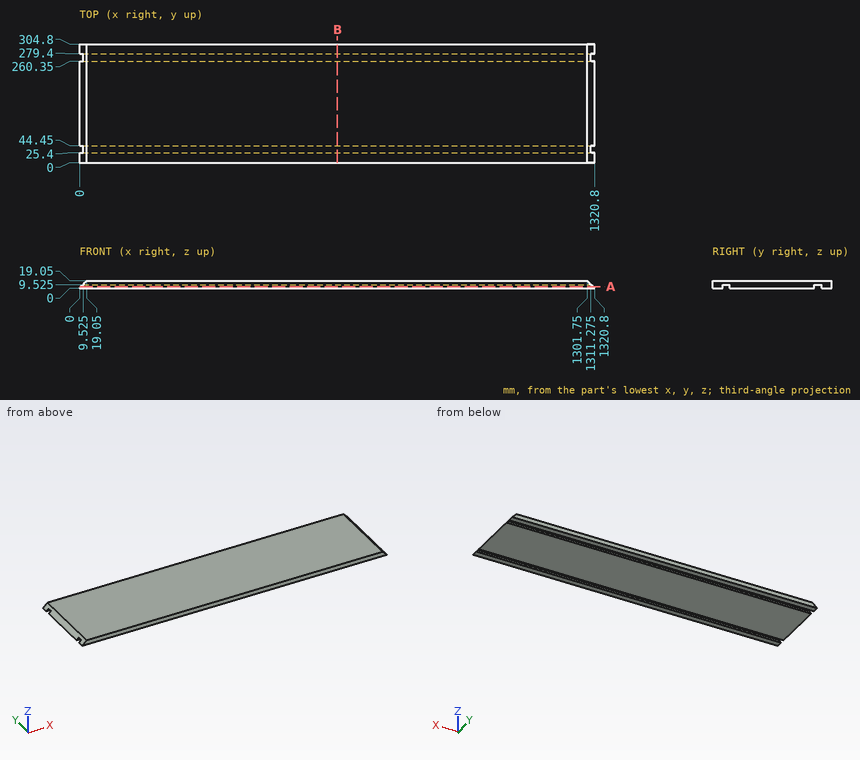
Print and shaded views of the part. All mm, measured from the part's lowest x, y and z. Give positions to 0.01 mm unless a question says otherwise; leave off trailing zeros. Loops run counter-clockwise (first coordinate to the right, second up) from the corner with the lowest first, then second, coordinate; pieces in that order, holes last.
1) Saw through at B-B (x = 661.5). Write the cut outline in (y, z) (3 decimals), plus the area to 3 significant figures.
2) Wall check: line 1 (Y direction, x = 846, z = 1.75); line 2 (X direction, y = 186.5, z = 9.75); line 3 (Z direction, x = 1073.5, y = 39) (3 decimals). Give the ranges that are in metal, low to high.
3) Flat gauge pins, fed straight in: pin 1 Ø3 at (y, z) = (77, 7.5) entering from -X; pin 2 Ø8 at (y, z) = (147.5, 11.5) entering from -X; pin 3 Ø5.5 at (x, y) = (665, 265.5) entering from -Z (3 decimals). Where does each tip first touch, or does it go through?
4) Saw through at A-A (z = 4.25). Write the cut outline in (x, y).
Answer block:
1. outline: (0, 0) - (25.4, 0) - (25.4, 9.525) - (44.45, 9.525) - (44.45, 0) - (260.35, 0) - (260.35, 9.525) - (279.4, 9.525) - (279.4, 0) - (304.8, 0) - (304.8, 19.05) - (0, 19.05) - close
1. area: 5,440 mm2
2. line 1: y = 0 to 25.4, 44.45 to 260.35, 279.4 to 304.8
2. line 2: x = 9.75 to 1311.05
2. line 3: z = 9.525 to 19.05
3. pin 1: stops at x = 6
3. pin 2: stops at x = 7.5
3. pin 3: stops at z = 9.525
4. outline: (4.25, 0) - (1316.55, 0) - (1316.55, 25.4) - (4.25, 25.4) - close; (4.25, 44.45) - (1316.55, 44.45) - (1316.55, 260.35) - (4.25, 260.35) - close; (4.25, 279.4) - (1316.55, 279.4) - (1316.55, 304.8) - (4.25, 304.8) - close
